```python
from build123d import *

# Parameters (mm, degrees)
SKETCH2_R                = 12
SKETCH2_R_2              = 10.8
CUT_EXTRUDE1_DEPTH       = 20
CUT_EXTRUDE1_DEPTH_BACK  = 20
SKETCH3_R                = 4.14257131
BOSS_EXTRUDE1_DEPTH      = 1
BOSS_EXTRUDE1_DEPTH_BACK = 1
SKETCH4_R                = 2.5


with BuildPart() as part:
    # Sweep1: sweep along a path in Sketch1
    with BuildLine(Plane.XY) as sweep1_path:
        Line((-209.367896725, 0), (41.706660839, 0))
        ThreePointArc((41.706660839, 0), (57.097567289, -2.713832065), (70.632103275, -10.52800006))
        Line((70.632103275, -10.52800006), (120.632103275, -52.482981619))
    # Sketch2 → Sweep1 (sweep)
    with BuildSketch(Plane(origin=(-209.367896725, 0, 0), x_dir=(0, 0, -1), z_dir=(1, 0, 0))):
        Circle(SKETCH2_R)
        Circle(SKETCH2_R_2, mode=Mode.SUBTRACT)
    sweep(path=sweep1_path.line)

    # Sketch3 → Cut-Extrude1 (cut, two sides: drawn at the far end of the back side and taken through both)
    with BuildSketch(Plane.XY.offset(-CUT_EXTRUDE1_DEPTH_BACK)):
        with Locations(Location((108.258660408, -42.100430272, 0), (0, 0, 180))):
            Circle(SKETCH3_R)
    extrude(amount=CUT_EXTRUDE1_DEPTH + CUT_EXTRUDE1_DEPTH_BACK, mode=Mode.SUBTRACT)

    # Sketch4 → Boss-Extrude1 (add, two sides: drawn at the far end of the back side and taken through both)
    # profile 1 of 2: a face of its own
    with BuildSketch(Plane.XY.offset(-BOSS_EXTRUDE1_DEPTH_BACK)):
        with BuildLine():
            Line((-128.741339592, 0), (-128.741339592, -37))
            ThreePointArc((-128.741339592, -37), (-118.741339592, -47), (-108.741339592, -37))
            Line((-108.741339592, -37), (-108.741339592, 0))
            Line((-108.741339592, 0), (-128.741339592, 0))
        make_face()
        with Locations((-118.741339592, -37)):
            Circle(SKETCH4_R, mode=Mode.SUBTRACT)
    # profile 2 of 2: a face of its own
    with BuildSketch(Plane.XY.offset(-BOSS_EXTRUDE1_DEPTH_BACK)):
        with BuildLine():
            Line((-24.741339592, 0), (-4.741339592, 0))
            Line((-4.741339592, 0), (-4.741339592, -37))
            ThreePointArc((-4.741339592, -37), (-14.741339592, -47), (-24.741339592, -37))
            Line((-24.741339592, -37), (-24.741339592, 0))
        make_face()
        with Locations((-14.741339592, -37)):
            Circle(SKETCH4_R, mode=Mode.SUBTRACT)
    extrude(amount=BOSS_EXTRUDE1_DEPTH + BOSS_EXTRUDE1_DEPTH_BACK)


solid = part.part
```
Design review of the part built by this model. Coordinates are the model's own, in mm. A direction names the side the tool comes from. Coordinates: 2 decimals unless noted, no trailing zeros. Order: outer loops, then holes, each group sorted by start corner. A loop starts at its lowest first (then second) coordinate and runs counter-clockwise, first axis right, second up. Notation, with made-up numbers: M 9.25,68 L 62.25,68 A30 cw 62.25,100 Z; hole C 36,45.25 d2. An arc over 180 degrees is marked long. Answer as a JSON object with one key per item and string values. Group by question number.
1) Add section C-C, the plane y = -22.5. Count the separate pieces of the cut face and the enclosed holes in it, then the cut area to 3 significant figures.
2) Mouldability with a two-part tool opening along X and no side actions: class faces 5 (the flat face through (-209.368, -5, -10)), 6 (the flat face through (-119, -5, 1)), 7 (the cylindrical face through (-14.521, -46.998, -0.014)) as pulls with the +X half, pulls with the -X half, needs draft (parallel to the pull), parting line crosses it, or undercut.
3) Wall thickness on L1, parallel to X at y = -22, z = 0; L2, parallel to Z at x = -18, y = -25; L3, parallel to Y at x = -66, z = -7.5: over which ranges is each line inside the solid? List them lowest first.
4) Add section B-B, the plane x = -181.5. Write out the cut boundary in (y, z), then the cut area to 3 significant figures.
5) Tool access review of faces 1 (the flat face through (-119, -29, 1)), 2 (the cylindrical face through (104.307, -43.345, -11.001)), 3 (the flat face through (-15, -5, -1)), 4 (the flat face through (-119, -29, -1)): name each direction out of +Z, -Z, +X, -X, +Y, -Y from which nothing blocks a thin tool from reaching the whole face with its end or side.
6) Add section A-A, the plane z = 5. Write out the cut boundary in (x, y).
7) For pin 1 (5 mm diameter, centred on x = -85.5, z = -6.5, fed in from +Y); pin 2 (22 mm diameter, centred on x = -12, y = -29.5, fed in from -Z); pin 3 (1.6 mm diameter, centred on y = -6.5, z = 0.5, fed in from -X), all flat-tipped, find the tip position at first contact; note any pin that passes through.
Computed values:
{
 "1": {"separate pieces": "3", "enclosed holes": "1", "area": "214 mm^2"},
 "2": {"face 5": "pulls with the -X half", "face 6": "needs draft", "face 7": "undercut"},
 "3": {"L1": "x = -128.74 to -108.74, -24.74 to -4.74, 65.64 to 67.5, 101.11 to 102.97", "L2": "z = -1 to 1", "L3": "y = -9.37 to -7.77, 7.77 to 9.37"},
 "4": {"outline": "C 0,0 d24; hole C 0,0 d21.6", "area": "86.0 mm^2"},
 "5": {"face 1": "+Z, -X, -Y", "face 2": "+Z, -Z", "face 3": "-X", "face 4": "-Z, -X, -Y"},
 "6": {"outline": "M -209.37,-10.91 L 41.71,-10.91 A34.09 cw 63.62,-18.88 L 113.62,-60.84 L 114.48,-59.82 L 64.48,-17.86 A35.43 ccw 41.71,-9.57 L -209.37,-9.57 Z; M -209.37,9.57 L 41.71,9.57 A54.57 cw 76.79,-3.19 L 126.79,-45.15 L 127.64,-44.13 L 77.64,-2.17 A55.91 ccw 41.71,10.91 L -209.37,10.91 Z"},
 "7": {"pin 1": "stops at y = 11.31", "pin 2": "stops at z = -1", "pin 3": "stops at x = -128.74"}
}
